Check sheet for the drawn part. Datum: minimum x, y, z corner. Units: mm. A direction names the side the tool comes from. Coordinates: 2 decimals unless noted, no trailing zeros. Order: outer loops, then holes, each group sorted by start corner. A loop starts at its lowest first (then second) coordinate and runs counter-clockwise, first axis right, second up. Notation, with made-up numbers: M -18.75,-21 L 36.25,-21 A14 cw 36.25,-15 Z; hole C -12,54.25 d7. An arc over 180 degrees is marked long. Return JSON: item names as keys, results as strings. Group by question number.
Q1. Thickness scan on probe 1 along Y at (x, z) = (36.15, 10); probe 2 along X at (y, z) = (2, 15); probe 3 along Y at (x, z) = (24, 13.5). Record the ranges inside material, lowest first.
Q2. Go/stop test with flat-tipped pins: pin 1 Ø5 at (y, z) = (29, 20) entering from -X; pin 2 Ø15 at (y, z) = (28, 8.5) entering from -X; pin 3 Ø4 at (x, z) = (14.5, 21.5) entering from -Y; pin 4 Ø6 at (x, z) = (6, 8.5) entering from +Y. Record where each tip stops, or that it passes through.
Q3. Section check C-C, the plane z = 15. Enter the section's corners in (x, y).
Q4. Section check B-B, the plane x = 17.5. Enter the section's corners in (y, z).
Q5. Section check D-D, the plane z = 20. Enter the section's corners in (x, y).
Q6. Section check A-A, the plane y = 9. Enter the section's corners in (x, z), then the cut area to 3 significant figures.
Q7. Mould release check, pull along Z, two halves, no side actions. Record for the marked faces 3 and 4: pulls with the +Z half, pulls with the -Z half, needs draft (parallel to the pull), parting line crosses it, or undercut.
Q8. Access from +Z, -Z, +X, -X, +Y, -Y to the whole of each face (thin tool, end or side, straight path). Record for the marked faces 1 and 2.
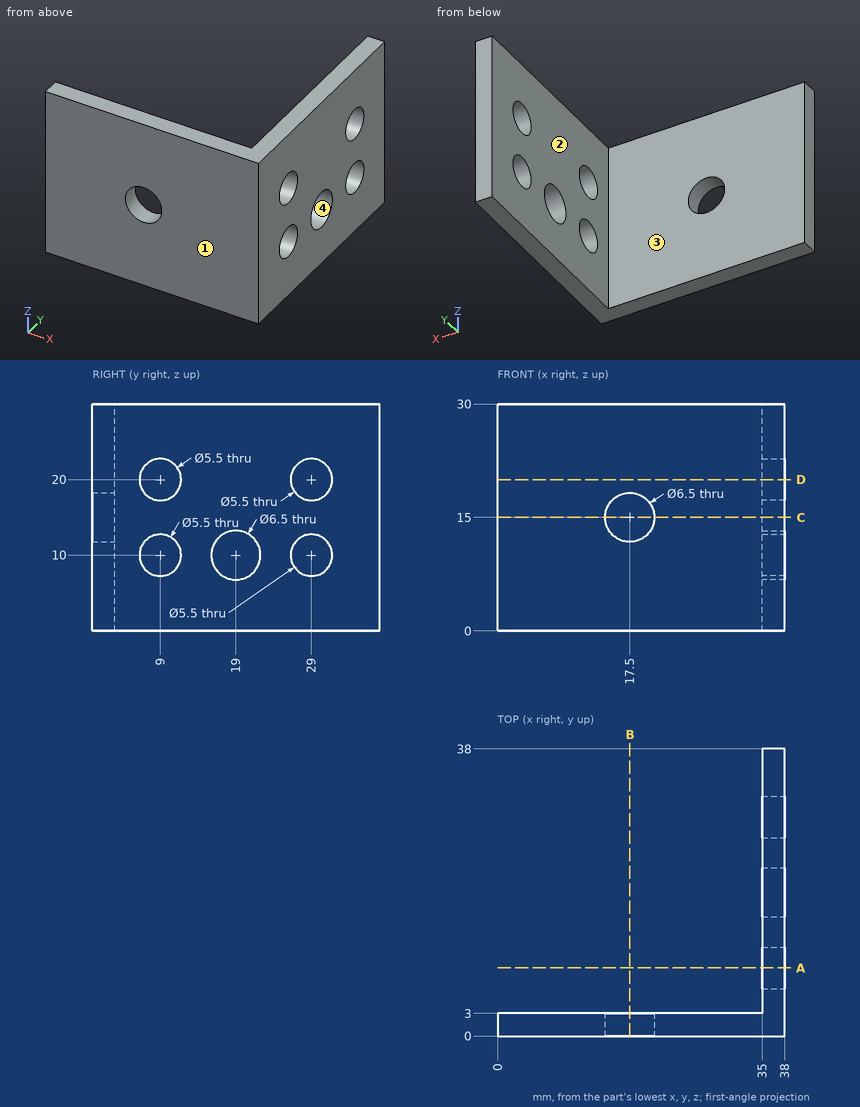
Numbers:
{
 "1": {"probe 1": "y = 0 to 6.25, 11.75 to 15.75, 22.25 to 26.25, 31.75 to 38", "probe 2": "x = 0 to 14.25, 20.75 to 38", "probe 3": "y = 0 to 3"},
 "2": {"pin 1": "passes through", "pin 2": "stops at x = 35", "pin 3": "stops at y = 0", "pin 4": "stops at y = 3"},
 "3": {"outline": "M 0,0 L 14.25,0 L 14.25,3 L 0,3 Z; M 20.75,0 L 38,0 L 38,38 L 35,38 L 35,3 L 20.75,3 Z"},
 "4": {"outline": "M 0,0 L 3,0 L 3,11.75 L 0,11.75 Z; M 0,18.25 L 3,18.25 L 3,30 L 0,30 Z"},
 "5": {"outline": "M 0,0 L 38,0 L 38,6.25 L 35,6.25 L 35,3 L 0,3 Z; M 35,11.75 L 38,11.75 L 38,26.25 L 35,26.25 Z; M 35,31.75 L 38,31.75 L 38,38 L 35,38 Z"},
 "6": {"outline": "M 35,0 L 38,0 L 38,7.25 L 35,7.25 Z; M 35,12.75 L 38,12.75 L 38,17.25 L 35,17.25 Z; M 35,22.75 L 38,22.75 L 38,30 L 35,30 Z", "area": "57.0 mm2"},
 "7": {"face 3": "needs draft", "face 4": "undercut"},
 "8": {"face 1": "+Z, -Z, +X, -X, -Y", "face 2": "+Z, -Z, -X, +Y"}
}
